Design review of the part built by this model. Coordinates are the model's own, in mm. Face numbers are marked on the shaded views. Coordinates: 2 decimals unless noted, no trailing zeros. Loops run counter-clockwise (first coordinate to the right, second up) from the corner with the lowest first, then second, coordinate; pieces in that order, holes last. Notation, with made-up numbers: M 42,66.25 L 86,66.25 A19 ccw 86,86.25 Z; hole C -22,70 d9. An arc over 180 degrees is marked long. Put each result on its own line as item: value. Start each with the question number.
(1) Clearance check with flat-ended pins moving along their axes: pin 1 (5.5 mm diameter, centred on x = 0, y = 0, fed in from -Z); pin 2 (1 mm diameter, centred on y = 4, z = 9.5, fed in from -X); pin 3 (2.5 mm diameter, centred on x = 9, y = -1.5, fed in from +Z). State where each tip first meets the part, or that it passes through.
(2) For probe 1 along Y at (x, z) = (0, 5.5); probe 2 along Z at (x, y) = (-1.25, -1.5); probe 3 along Y at (x, z) = (0, 11.25) (3 decimals), list the stretches that pass through material, from the lowest coordinate up. Write a range as [from, to].
(3) Take a section at A-A, the plane z = 3.75. Give the boundary of the cut face in (x, y).
(4) The part is to be moulded in two halves that separate along Y. For the marked faces 1, 2 and 3, say which applies: +Y half, -Y half, draft (parallel to the pull), parting line (faces both ways), or undercut.
```python
from build123d import *

# Parameters (mm, degrees)
F0_R     = 3.5
F1_DEPTH = 6
F2_R     = 8.6602540378
F3_DEPTH = 6
F4_R     = 5.99999
F6_DEPTH = 3
F5_R     = 0.75
F7_DEPTH = 12.001


# Not quite as in the source:
# - a fillet or chamfer is up to 0.001 mm smaller than in the source, because OpenCascade refuses the exact size


with BuildPart() as f1:
    # F0 (on Top) → F1 (new body)
    with BuildSketch(Plane.XY):
        Polygon((5, 8.6602540378), (-5, 8.6602540378), (-10, 0), (-5, -8.6602540378), (5, -8.6602540378), (10, 0), align=None)
        Circle(F0_R, mode=Mode.SUBTRACT)
    extrude(amount=F1_DEPTH)

    # F2 (on face) → F3 (join)
    with BuildSketch(Plane.XY.offset(6)):
        Circle(F2_R)
    extrude(amount=F3_DEPTH)

    # F4 (radius 6 in the source; OpenCascade refuses exactly that, so slightly less here)
    f4_edges = [f1.edges().sort_by_distance(p)[0] for p in [
        (-8.660254, 0, 12),
    ]]
    fillet(f4_edges, radius=F4_R)

    # F6 (cut): a face of the model
    f6_faces = [f1.faces().sort_by_distance(p)[0] for p in [
        (0, 0, 6),
    ]]
    extrude(f6_faces, amount=-F6_DEPTH, mode=Mode.SUBTRACT)

    # F5 (on face) → F7 (cut, through all)
    with BuildSketch(Plane.XY.offset(12)):
        Circle(F5_R)
    extrude(amount=-F7_DEPTH, mode=Mode.SUBTRACT)


solid = f1.part
```
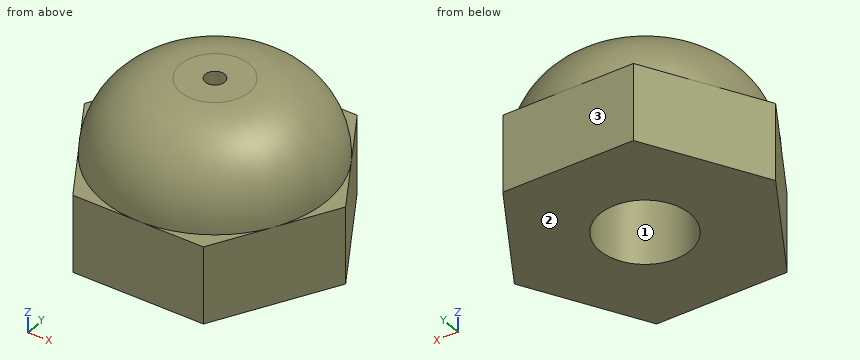
Computed values:
1. pin 1: stops at z = 9
1. pin 2: stops at x = -6.86
1. pin 3: stops at z = 8.97
2. probe 1: y = [-8.66, -3.5], [3.5, 8.66]
2. probe 2: z = [9, 12]
2. probe 3: y = [-5.565, -0.75], [0.75, 5.565]
3. outline: M -10,0 L -5,-8.66 L 5,-8.66 L 10,0 L 5,8.66 L -5,8.66 Z; hole C 0,0 d7
4. face 1: undercut
4. face 2: draft
4. face 3: +Y half
